```python
from build123d import *

# Parameters (mm, degrees)
ESBO_O1_R                = 1.75
RESSALTO_EXTRUS_O1_DEPTH = 6.5
CORTE_EXTRUS_O1_DEPTH    = 3.5
CORTE_EXTRUS_O2_DEPTH    = 4.5
ESBO_O3_3_R              = 4.25
CORTE_EXTRUS_O3_DEPTH    = 33.30325061
ESBO_O4_R                = 5.75
ESBO_O4_R_2              = 4.25
RESSALTO_EXTRUS_O2_DEPTH = 1
CHANFRO1_SIZE            = 1
FILETE1_R                = 3


# Some blends are built 0.0001 mm under size
with BuildPart() as part:
    # Esboço1 → Ressalto-extrusão1 (new body)
    with BuildSketch(Plane.XY):
        with BuildLine():
            Line((-11.5, -6), (11.5, -6))
            ThreePointArc((11.5, -6), (15.035533906, -4.535533906), (16.5, -1))
            Line((16.5, -1), (16.5, 22))
            ThreePointArc((16.5, 22), (15.035533906, 25.535533906), (11.5, 27))
            Line((11.5, 27), (-11.5, 27))
            ThreePointArc((-11.5, 27), (-15.035533906, 25.535533906), (-16.5, 22))
            Line((-16.5, 22), (-16.5, -1))
            ThreePointArc((-16.5, -1), (-15.035533906, -4.535533906), (-11.5, -6))
        make_face()
        with Locations(Location((0, 0, 0), (0, 0, 180))):
            Circle(ESBO_O1_R, mode=Mode.SUBTRACT)
        with Locations(Location((-10.5, 21, 0), (0, 0, 180))):
            Circle(ESBO_O1_R, mode=Mode.SUBTRACT)
        with Locations(Location((10.5, 21, 0), (0, 0, 180))):
            Circle(ESBO_O1_R, mode=Mode.SUBTRACT)
    extrude(amount=RESSALTO_EXTRUS_O1_DEPTH)

    # Esboço2 → Corte-extrusão1 (cut)
    with BuildSketch(Plane.XY.offset(6.5)):
        Polygon((-12.174315781, 18.1), (-8.825684219, 18.1), (-7.151368439, 21), (-8.825684219, 23.9), (-12.174315781, 23.9), (-13.848631561, 21), align=None)
        Polygon((8.825684219, 18.1), (12.174315781, 18.1), (13.848631561, 21), (12.174315781, 23.9), (8.825684219, 23.9), (7.151368439, 21), align=None)
        Polygon((-1.674315781, 2.9), (-3.348631561, 0), (-1.674315781, -2.9), (1.674315781, -2.9), (3.348631561, 0), (1.674315781, 2.9), align=None)
    extrude(amount=-CORTE_EXTRUS_O1_DEPTH, mode=Mode.SUBTRACT)

    # Esboço3 → Corte-extrusão2 (cut)
    with BuildSketch(Plane(origin=(0, 0, 0), x_dir=(-1, 0, 0), z_dir=(0, 0, -1))):
        Polygon((3.897114317, 17.25), (-3.897114317, 17.25), (-7.794228634, 10.5), (-3.897114317, 3.75), (3.897114317, 3.75), (7.794228634, 10.5), align=None)
    extrude(amount=-CORTE_EXTRUS_O2_DEPTH, mode=Mode.SUBTRACT)

    # Esboço3<3> → Corte-extrusão3 (cut, through all)
    with BuildSketch(Plane(origin=(0, 0, 0), x_dir=(-1, 0, 0), z_dir=(0, 0, -1))):
        with Locations((0, 10.5)):
            Circle(ESBO_O3_3_R)
    extrude(amount=-CORTE_EXTRUS_O3_DEPTH, mode=Mode.SUBTRACT)

    # Esboço4 → Ressalto-extrusão2 (add)
    with BuildSketch(Plane.XY.offset(6.5)):
        with Locations((0, 10.5)):
            Circle(ESBO_O4_R)
        with Locations(Location((0, 10.5, 0), (0, 0, 180))):
            Circle(ESBO_O4_R_2, mode=Mode.SUBTRACT)
    extrude(amount=RESSALTO_EXTRUS_O2_DEPTH)

    # Chanfro1
    chanfro1_edges = [part.edges().sort_by_distance(p)[0] for p in [
        (-5.75, 10.5, 7.5),
    ]]
    chamfer(chanfro1_edges, length=CHANFRO1_SIZE - 0.0001)  # a hair under: the kernel refuses the full size

    # Filete1
    # the kernel refuses this fillet: 3 mm, written as the material it takes off along each edge
    with BuildSketch(Plane(origin=(11.5, 22, 6.5), x_dir=(1, 0, 0), z_dir=(0, -1, 0))) as filete1_piece_1:
        with BuildLine():
            CenterArc((5 - FILETE1_R, -FILETE1_R), FILETE1_R, 0, 90)
            Line((5, -FILETE1_R), (5, 0))
            Line((5, 0), (5 - FILETE1_R, 0))
        make_face()
    revolve(axis=Axis((11.5, 22, 6.5), (0, 0, 1)), revolution_arc=90, mode=Mode.SUBTRACT)
    with BuildSketch(Plane(origin=(11.5, 27, 6.5), x_dir=(0, -1, 0), z_dir=(-1, 0, 0)), Plane(origin=(-16.5, 22, 6.5), x_dir=(1, 0, 0), z_dir=(0, -1, 0)), Plane(origin=(-11.5, -6, 6.5), x_dir=(0, 1, 0), z_dir=(1, 0, 0)), Plane(origin=(16.5, -1, 6.5), x_dir=(-1, 0, 0), z_dir=(0, 1, 0))) as filete1_piece_2:
        with BuildLine():
            CenterArc((FILETE1_R, -FILETE1_R), FILETE1_R, 90, 90)
            Line((0, -FILETE1_R), (0, 0))
            Line((0, 0), (FILETE1_R, 0))
        make_face()
    extrude(amount=23, mode=Mode.SUBTRACT)
    with BuildSketch(Plane(origin=(-11.5, 22, 6.5), x_dir=(0, 1, 0), z_dir=(1, 0, 0))) as filete1_piece_3:
        with BuildLine():
            CenterArc((5 - FILETE1_R, -FILETE1_R), FILETE1_R, 0, 90)
            Line((5, -FILETE1_R), (5, 0))
            Line((5, 0), (5 - FILETE1_R, 0))
        make_face()
    revolve(axis=Axis((-11.5, 22, 6.5), (0, 0, 1)), revolution_arc=90, mode=Mode.SUBTRACT)
    with BuildSketch(Plane(origin=(-11.5, -1, 6.5), x_dir=(-1, 0, 0), z_dir=(0, 1, 0))) as filete1_piece_4:
        with BuildLine():
            CenterArc((5 - FILETE1_R, -FILETE1_R), FILETE1_R, 0, 90)
            Line((5, -FILETE1_R), (5, 0))
            Line((5, 0), (5 - FILETE1_R, 0))
        make_face()
    revolve(axis=Axis((-11.5, -1, 6.5), (0, 0, 1)), revolution_arc=90, mode=Mode.SUBTRACT)
    with BuildSketch(Plane(origin=(11.5, -1, 6.5), x_dir=(0, -1, 0), z_dir=(-1, 0, 0))) as filete1_piece_5:
        with BuildLine():
            CenterArc((5 - FILETE1_R, -FILETE1_R), FILETE1_R, 0, 90)
            Line((5, -FILETE1_R), (5, 0))
            Line((5, 0), (5 - FILETE1_R, 0))
        make_face()
    revolve(axis=Axis((11.5, -1, 6.5), (0, 0, 1)), revolution_arc=90, mode=Mode.SUBTRACT)


solid = part.part
```
CAD build for the part. Positions are in the model's coordinates, mm. A direction names the side the tool comes from. Round coordinates to 2 decimals unless told otherwise and drop trailing zeros. Loops run counter-clockwise (first coordinate to the right, second up) from the corner with the lowest first, then second, coordinate; pieces in that order, holes last. Notation, with made-up numbers: M -0.5,-15 L 55.5,-15 A17 cw 55.5,-7 Z; hole C 1,46.5 d4. An arc over 180 degrees is marked long. Use a Markdown table: item, result. Add a question column.
(1) Pull direction X, two halves, no side cores. Call faces 1 (the face through (0, 27, 2)), 2 (the face through (-10, 23.9, 5)), 3 (the face through (-15.07, -4.5, 1.73)): +X half, -X half, draft (parallel to the pull), parting line (faces both ways), or undercut.
(2) Cut at D-D (y = 0.5). Give the cut face in (x, z), and give its area (3 significant figures).
(3) Flat gauge pins, fed straight in: pin 1 (1.1 mm diameter, centred on x = -12.5, y = 22.5, fed in from +Z); pin 2 (1.5 mm diameter, centred on x = 2.5, z = 6, fed in from -Y); pin 3 (3 mm diameter, centred on x = 1, y = -1, fed in from +Z); pin 4 (2.5 mm diameter, centred on x = -0.5, z = 4, fed in from -Y). Where does each tip first touch, or does it go through?
(4) Which spindle directions (+Z, -Z, +X, -X, +Y, -Y) get a long thin tool onto all of the face, cutting with end or side? Do faces 4 (the face through (8, 22.47, 4.77)), 5 (the face through (0.16, 26.1, 5.64)), 6 (the face through (5.82, 13.92, 2.22)). Say none if no direction does.
(5) Drill centre lines: line 1 (X direction, y = 21, z = 1.2); line 2 (Y direction, x = 0, z = 2.45); line 3 (Y direction, x = 11, z = 3.5). Where is each one in solid material? Low to high.
(6) Cut at C-C (x = 0). State how many separate pieces and enclosed holes the cut face has, and give its area (3 significant figures).
(7) Cut at B-B (x = -10.5). Give the cut face in (y, z).
(8) Cut at A-A (z = 0.75). Give the cut face in (x, y).
Geometry says:
| question | item | result |
|---|---|---|
| 1 | face 1 | draft |
| 1 | face 2 | undercut |
| 1 | face 3 | -X half |
| 2 | outline | M -16.5,0 L -1.68,0 L -1.68,3 L -3.06,3 L -3.06,6.5 L -13.5,6.5 A3 ccw -16.5,3.5 Z; M 1.68,0 L 16.5,0 L 16.5,3.5 A3 ccw 13.5,6.5 L 3.06,6.5 L 3.06,3 L 1.68,3 Z |
| 2 | area | 179 mm² |
| 3 | pin 1 | stops at z = 6.5 |
| 3 | pin 2 | stops at y = -5.44 |
| 3 | pin 3 | stops at z = 3 |
| 3 | pin 4 | stops at y = -6 |
| 4 | face 4 | +Z |
| 4 | face 5 | +Z, +X, -X, +Y |
| 4 | face 6 | -Z |
| 5 | line 1 | x = -16.5 to -12.25, -8.75 to 8.75, 12.25 to 16.5 |
| 5 | line 2 | y = -6 to -1.75, 1.75 to 3.75, 17.25 to 27 |
| 5 | line 3 | y = -6 to 18.1, 23.9 to 27 |
| 6 | separate pieces | 3 |
| 6 | enclosed holes | 0 |
| 6 | area | 104 mm² |
| 7 | outline | M -6,0 L 19.25,0 L 19.25,3 L 18.1,3 L 18.1,6.5 L -3,6.5 A3 ccw -6,3.5 Z; M 22.75,0 L 27,0 L 27,3.5 A3 ccw 24,6.5 L 23.9,6.5 L 23.9,3 L 22.75,3 Z |
| 8 | outline | M -16.5,-1 A5 ccw -11.5,-6 L 11.5,-6 A5 ccw 16.5,-1 L 16.5,22 A5 ccw 11.5,27 L -11.5,27 A5 ccw -16.5,22 Z; hole C -10.5,21 d3.5; hole M -7.79,10.5 L -3.9,3.75 L 3.9,3.75 L 7.79,10.5 L 3.9,17.25 L -3.9,17.25 Z; hole C 0,0 d3.5; hole C 10.5,21 d3.5 |
